Work out the finished part from the listing and answer in its coordinate system (mm). Face numbers are marked on the shaded views. A direction names the side the tool comes from. Round coordinates to 2 decimals unless told otherwise and drop trailing zeros. Order: outer loops, then holes, each group sorted by start corner. A loop starts at its lowest first (then second) coordinate and runs counter-clockwise, first axis right, second up. Notation, with made-up numbers: (54.25, 20) -> (66.25, 20) arc R25 cw to (66.25, 49) -> close; hole circle Ø4 at (-32, 79). An arc over 180 degrees is marked (long way). Use a Markdown table: item, result. Add a question column.
Item 1: Flat-ended cylindrical pins translate along their axes: P1, Ø5, axis at y = -29.02, z = 10.03, coming from the +X side; P2, Ø3.5, axis at y = 41.98, z = 10.03, coming from the -X side; P3, Ø5.5, axis at x = 1, z = 2.5, coming from the +Y side; P4, Ø12.5, axis at x = 2, y = -5, coming from the +Z side. Find the tip coordinate at first contact, or state that the pin passes through.
Item 2: For a pull along Y with two mould halves and no side action, classify the marked faces 1, 2, 3 and 4 as +Y half, -Y half, draft (parallel to the pull), parting line (faces both ways), or undercut.
Item 3: A cutting plane is placed at D-D, the plane z = 6.5. Determine the outline of the cut face in (x, y).
Item 4: A cutting plane is placed at A-A, the plane y = -4.25. Determine the outline of the cut face in (x, z), plus the area to 3 significant figures.
Item 5: A cutting plane is placed at C-C, the plane x = -4.5. Determine the outline of the cut face in (y, z), plus the area to 3 significant figures.
Item 6: Find the intervals of material crossed by L1, parallel to X at y = -4.25, z = 1.15; L2, parallel to X at y = 4.25, z = 3.5; L3, parallel to Y at x = 7.75, z = 3.1, in increasing order. Write a range as [from, to].
Item 7: A cutting plane is placed at B-B, the plane y = 4.25. Determine the outline of the cut face in (x, z).
Item 8: A tool of negligible diameter and unlimited length cuts with its end or side. For the marked faces 5, 6, 7 and 8, from which of +Z, -Z, +X, -X, +Y, -Y can it reach the whole face along a straight path? Write none if from no direction.
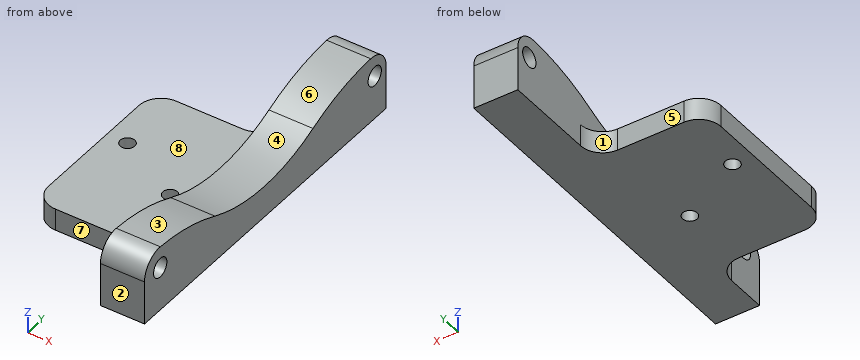
from build123d import *

# Parameters (mm, degrees)
F0_W     = 25
F0_H     = 40
F1_DEPTH = 5
F2_D     = 3.3
F3_DEPTH = 15
F5_DEPTH = 100
F6_R     = 40
F7_DEPTH = 25
F8_R     = 5
F9_R     = 50
F11_D    = 4.4
F12_R    = 5


with BuildPart() as f1:
    # F0 (on Top) → F1 (new body)
    with BuildSketch(Plane.XY):
        Rectangle(F0_W, F0_H)
    extrude(amount=F1_DEPTH)

    # F2 (through all)
    with Locations(Plane(origin=(0, 0, 0), x_dir=(1, 0, 0), z_dir=(0, 0, -1))):
        with Locations((-7.75, -4.25), (7.75, 4.25)):
            Hole(F2_D / 2)

    # F0 (on Top) → F3 (join)
    with BuildSketch(Plane.XY):
        Polygon((12.5, 45.7778535783), (12.5, 20), (12.5, -20), (12.5, -34.2221464217), (22.5, -34.2221464217), (22.5, 45.7778535783), align=None)
    extrude(amount=F3_DEPTH)

    # F4 (on face) → F5 (cut)
    with BuildSketch(Plane.XZ.offset(34.2221464217)):
        Polygon((24.4068726897, 16.530605033), (15.8845428377, 16.530605033), (15.8845428377, 15), (22.5, 15), (22.5, 0), (15.8845428377, 0), (15.8845428377, -1.5078758588), (24.4068726897, -1.5078758588), align=None)
    extrude(amount=-F5_DEPTH, mode=Mode.SUBTRACT)

    # F6 (on Right) → F7 (cut)
    with BuildSketch(Plane.YZ):
        with Locations((5.292929709, 47.2443401814)):
            Circle(F6_R)
    extrude(amount=F7_DEPTH, mode=Mode.SUBTRACT)

    # F8
    f8_edges = [f1.edges().sort_by_distance(p)[0] for p in [
        (12.5, -20, 2.5),
        (12.5, 20, 2.5),
        (-12.5, 20, 2.5),
        (-12.5, -20, 2.5),
    ]]
    fillet(f8_edges, radius=F8_R)

    # F9
    f9_edges = [f1.edges().sort_by_distance(p)[0] for p in [
        (17.5, -18.377781, 15),
        (17.5, 28.96364, 15),
    ]]
    fillet(f9_edges, radius=F9_R)

    # F11 (through all)
    with Locations(Plane.YZ.offset(22.5)):
        with Locations((-29.0194526315, 10.0306486711), (41.9805473685, 10.0306486711)):
            Hole(F11_D / 2)

    # F12
    f12_edges = [f1.edges().sort_by_distance(p)[0] for p in [
        (17.5, -34.222146, 15),
        (17.5, 45.777854, 15),
    ]]
    fillet(f12_edges, radius=F12_R)


solid = f1.part
Reported:
| question | item | result |
|---|---|---|
| 1 | P1 | x = 22.5 |
| 1 | P2 | through |
| 1 | P3 | y = 20 |
| 1 | P4 | z = 5 |
| 2 | face 1 | +Y half |
| 2 | face 2 | -Y half |
| 2 | face 3 | undercut |
| 2 | face 4 | undercut |
| 3 | outline | (12.5, -34.22) -> (22.5, -34.22) -> (22.5, 45.78) -> (12.5, 45.78) -> close |
| 4 | outline | (-12.5, 0) -> (6.1, 0) -> (6.1, 5) -> (-12.5, 5) -> close; (9.4, 0) -> (22.5, 0) -> (22.5, 8.4) -> (12.5, 8.4) -> (12.5, 5) -> (9.4, 5) -> close |
| 4 | area | 192 mm² |
| 5 | outline | (-20, 0) -> (20, 0) -> (20, 5) -> (-20, 5) -> close |
| 5 | area | 200 mm² |
| 6 | L1 | [-12.5, 6.1], [9.4, 22.5] |
| 6 | L2 | [-12.5, -9.4], [-6.1, 22.5] |
| 6 | L3 | [-20.01, -5.9], [-2.6, 20.01] |
| 7 | outline | (-12.5, 0) -> (-9.4, 0) -> (-9.4, 5) -> (-12.5, 5) -> close; (-6.1, 0) -> (22.5, 0) -> (22.5, 7.26) -> (12.5, 7.26) -> (12.5, 5) -> (-6.1, 5) -> close |
| 8 | face 5 | +Z, -Z, -X, +Y |
| 8 | face 6 | +Z, +X, -X |
| 8 | face 7 | +Z, -Z, -X, -Y |
| 8 | face 8 | +Z, -X, +Y, -Y |
